Part model, mm, in its own coordinate system. A direction names the side the tool comes from. Give positions to 0.01 mm unless a question says otherwise; leave off trailing zeros. Order: outer loops, then holes, each group sorted by start corner. A loop starts at its lowest first (then second) coordinate and runs counter-clockwise, first axis right, second up. Notation, with made-up numbers: (-37.75, -17.75) - (-17.75, -17.75) arc R21 cw to (-17.75, -12.75) - close; hole circle Ø11 at (12, -16). An arc over 180 degrees is marked (long way). One line per item, written item: value.
```python
from build123d import *

# Parameters (mm, degrees)
RESSALTO_EXTRUS_O1_DEPTH = 10
CORTE_EXTRUS_O1_REACH    = 44.778
ESBO_O2_R                = 1.6
FILETE1_R                = 1.5
FILETE2_R                = 1.5
FILETE3_R                = 1.5


# Some blends are built 0.0001 mm under size
with BuildPart() as part:
    # Esboço1 → Ressalto-extrusão1 (new body)
    with BuildSketch(Plane.XY):
        Polygon((-37, -3), (-20, -3), (-20, 0), (-31, 0), (-31, 13), (31, 13), (31, 0), (20, 0), (20, -3), (37, -3), (37, 19), (-37, 19), align=None)
    extrude(amount=RESSALTO_EXTRUS_O1_DEPTH)

    # Esboço2 → Corte-extrusão1 (cut, up to next)
    with BuildSketch(Plane(origin=(0, 0, 0), x_dir=(1, 0, 0), z_dir=(0, 1, 0)), mode=Mode.PRIVATE) as corte_extrus_o1_sk1:
        with Locations(Location((-25.5, -5, 0), (0, 0, 180))):
            Circle(ESBO_O2_R)
    corte_extrus_o1_tool1 = extrude(corte_extrus_o1_sk1.sketch, amount=-CORTE_EXTRUS_O1_REACH, mode=Mode.PRIVATE) & part.part
    # Esboço2 → Corte-extrusão1 (cut, up to next)
    with BuildSketch(Plane(origin=(0, 0, 0), x_dir=(1, 0, 0), z_dir=(0, 1, 0)), mode=Mode.PRIVATE) as corte_extrus_o1_sk2:
        with Locations(Location((25.5, -5, 0), (0, 0, 270))):
            Circle(ESBO_O2_R)
    corte_extrus_o1_tool2 = extrude(corte_extrus_o1_sk2.sketch, amount=-CORTE_EXTRUS_O1_REACH, mode=Mode.PRIVATE) & part.part
    add(corte_extrus_o1_tool1.solids().sort_by_distance((-25.5, 0, 5))[0], mode=Mode.SUBTRACT)
    add(corte_extrus_o1_tool2.solids().sort_by_distance((25.5, 0, 5))[0], mode=Mode.SUBTRACT)

    # Filete1
    filete1_edges = [part.edges().sort_by_distance(p)[0] for p in [
        (0, 19, 0),
        (0, 13, 0),
        (0, 13, 10),
        (0, 19, 10),
    ]]
    fillet(filete1_edges, radius=FILETE1_R)

    # Filete2
    filete2_edges = [part.edges().sort_by_distance(p)[0] for p in [
        (37, 7.25, 10),
        (37, 18.560660172, 9.560660172),
        (37, 7.25, 0),
        (37, 18.560660172, 0.439339828),
        (-37, 7.25, 10),
        (-37, 18.560660172, 9.560660172),
        (-37, 7.25, 0),
        (-37, 18.560660172, 0.439339828),
        (37, 19, 5),
        (-37, 19, 5),
        (-20, -3, 5),
        (20, -3, 5),
        (-20, 0, 5),
        (20, 0, 5),
        (31, 0, 5),
        (-31, 0, 5),
        (-37, -3, 5),
        (37, -3, 5),
    ]]
    fillet(filete2_edges, radius=FILETE2_R - 0.0001)  # a hair under: the kernel refuses the full size

    # Filete3
    # the kernel refuses this fillet: 1.5 mm, written as the material it adds along each edge
    with BuildSketch(Plane(origin=(31, 13, 1.5), x_dir=(0, -1, 0), z_dir=(0, 0, 1))) as filete3_piece_1:
        with BuildLine():
            CenterArc((FILETE3_R, -FILETE3_R), FILETE3_R, 90, 90)
            Line((0, -FILETE3_R), (0, 0))
            Line((0, 0), (FILETE3_R, 0))
        make_face()
    extrude(amount=7)
    with BuildSketch(Plane(origin=(-31, 13, 1.5), x_dir=(0, -1, 0), z_dir=(0, 0, 1))) as filete3_piece_2:
        with BuildLine():
            CenterArc((FILETE3_R, FILETE3_R), FILETE3_R, 180, 90)
            Line((0, FILETE3_R), (0, 0))
            Line((0, 0), (FILETE3_R, 0))
        make_face()
    extrude(amount=7)
    with BuildSketch(Plane(origin=(31, 14.5, 8.5), x_dir=(0, 0.5976672776328287, -0.8017442392976475), z_dir=(0, -0.8017442392976475, -0.5976672776328287))) as filete3_piece_3_section:
        with BuildLine():
            CenterArc((1.5 + FILETE3_R, -FILETE3_R), FILETE3_R, 90, 90)
            Line((1.5, -FILETE3_R), (1.5, 0))
            Line((1.5, 0), (1.5 + FILETE3_R, 0))
        make_face()
    filete3_piece_3 = revolve(axis=Axis((31, 14.5, 8.5), (1, 0, 0)), revolution_arc=233.296989237, mode=Mode.PRIVATE)
    filete3_piece_3 = split(filete3_piece_3, bisect_by=Plane(origin=(30.532557549, 13.375091575, 10), z_dir=(0, 0, -1)), keep=Keep.TOP, mode=Mode.PRIVATE)
    add(filete3_piece_3)
    with BuildSketch(Plane(origin=(-31, 14.5, 8.5), x_dir=(0, 0.5976672776328287, -0.8017442392976475), z_dir=(0, -0.8017442392976475, -0.5976672776328287))) as filete3_piece_4_section:
        with BuildLine():
            CenterArc((1.5 + FILETE3_R, FILETE3_R), FILETE3_R, 180, 90)
            Line((1.5, FILETE3_R), (1.5, 0))
            Line((1.5, 0), (1.5 + FILETE3_R, 0))
        make_face()
    filete3_piece_4 = revolve(axis=Axis((-31, 14.5, 8.5), (1, 0, 0)), revolution_arc=233.296989237, mode=Mode.PRIVATE)
    filete3_piece_4 = split(filete3_piece_4, bisect_by=Plane(origin=(-30.532557659, 13.37509149, 10), z_dir=(0, 0, -1)), keep=Keep.TOP, mode=Mode.PRIVATE)
    add(filete3_piece_4)
    with BuildSketch(Plane(origin=(31, 14.5, 1.5), x_dir=(0, 0.5976672776328277, 0.8017442392976482), z_dir=(0, -0.8017442392976482, 0.5976672776328277))) as filete3_piece_5_section:
        with BuildLine():
            CenterArc((1.5 + FILETE3_R, FILETE3_R), FILETE3_R, 180, 90)
            Line((1.5, FILETE3_R), (1.5, 0))
            Line((1.5, 0), (1.5 + FILETE3_R, 0))
        make_face()
    filete3_piece_5 = revolve(axis=Axis((31, 14.5, 1.5), (-1, 0, 0)), revolution_arc=233.296989237, mode=Mode.PRIVATE)
    filete3_piece_5 = split(filete3_piece_5, bisect_by=Plane(origin=(30.532557549, 13.375091575, 0), z_dir=(0, 0, 1)), keep=Keep.TOP, mode=Mode.PRIVATE)
    add(filete3_piece_5)
    with BuildSketch(Plane(origin=(-31, 14.5, 1.5), x_dir=(0, 0.5976672776328277, 0.8017442392976482), z_dir=(0, -0.8017442392976482, 0.5976672776328277))) as filete3_piece_6_section:
        with BuildLine():
            CenterArc((1.5 + FILETE3_R, -FILETE3_R), FILETE3_R, 90, 90)
            Line((1.5, -FILETE3_R), (1.5, 0))
            Line((1.5, 0), (1.5 + FILETE3_R, 0))
        make_face()
    filete3_piece_6 = revolve(axis=Axis((-31, 14.5, 1.5), (-1, 0, 0)), revolution_arc=233.296989237, mode=Mode.PRIVATE)
    filete3_piece_6 = split(filete3_piece_6, bisect_by=Plane(origin=(-30.532557571, 13.375091573, 0), z_dir=(0, 0, 1)), keep=Keep.TOP, mode=Mode.PRIVATE)
    add(filete3_piece_6)


solid = part.part
```
1) Cut at A-A, the plane x = 25.5. Give the cut face in (y, z).
Outcome:
outline: (-3, 0) - (0, 0) - (0, 3.4) - (-3, 3.4) - close; (-3, 6.6) - (0, 6.6) - (0, 10) - (-3, 10) - close; (13, 1.5) arc R1.5 ccw to (14.5, 0) - (17.5, 0) arc R1.5 ccw to (19, 1.5) - (19, 8.5) arc R1.5 ccw to (17.5, 10) - (14.5, 10) arc R1.5 ccw to (13, 8.5) - close
2) Cut at B-B, the plane y = 8.75. Give the cut face in (x, z).
Outcome:
outline: (-37, 1.5) arc R1.5 ccw to (-35.5, 0) - (-31, 0) - (-31, 10) - (-35.5, 10) arc R1.5 ccw to (-37, 8.5) - close; (31, 0) - (35.5, 0) arc R1.5 ccw to (37, 1.5) - (37, 8.5) arc R1.5 ccw to (35.5, 10) - (31, 10) - close
3) Cut at C-C, the plane z = 5. Give the number of separate pieces and of enclosed holes in the cut face, then the cut area to 3 significant figures.
Outcome:
separate pieces: 3
enclosed holes: 0
area: 681 mm^2
4) Cut at D-D, the plane x = -18. Give the cut face in (y, z).
Outcome:
outline: (13, 1.5) arc R1.5 ccw to (14.5, 0) - (17.5, 0) arc R1.5 ccw to (19, 1.5) - (19, 8.5) arc R1.5 ccw to (17.5, 10) - (14.5, 10) arc R1.5 ccw to (13, 8.5) - close
5) Pin check, flat tips, straight feed: pin 1 (1 mm diameter, centred on x = 16.5, z = 4, fed in from -Y); pin 2 (5 mm diameter, centred on x = -3, y = 11, fed in from +Z); pin 3 (8 mm diameter, centred on x = 7.5, y = 14, fed in from +Z). Stop position of each tip, or through.
Outcome:
pin 1: stops at y = 13
pin 2: stops at z = 9.62
pin 3: stops at z = 10
6) Drill centre lines: line 1 along X through (y, z) = (11.25, 5); line 2 along Y through (x, z) = (22, 4.5); line 3 along Z through (x, y) = (-25.5, -1.2). Where is each one in solid material? Low to high. Write a range as from..to.
Outcome:
line 1: x = -37..-31, 31..37
line 2: y = -3..0, 13..19
line 3: z = 0..3.4, 6.6..10
7) Which spindle directions (+Z, -Z, +X, -X, +Y, -Y) get a long thin tool onto all of the face, cutting with end or side? Do faces 5 (the cylindrical face through (0.41, 13.45, 9.57)), 6 (the cylindrical face through (-30.55, 0.43, 5.07)), 7 (the flat face through (-29, -3, 5)), 8 (the cylindrical face through (20.45, -2.57, 5.07)), 9 (the cylindrical face through (25.981, -1.479, 6.526)). Say none if no direction does.
Outcome:
face 5: +Z
face 6: +Z, -Z
face 7: +Z, -Z, +X, -X, -Y
face 8: +Z, -Z, -Y
face 9: -Y
8) Mould opens along X. For faces 1 (the cylindrical face through (-0.5, 18.55, 0.43)), 2 (the cylindrical face through (-36.57, 7.39, 0.45)), 3 (the cylindrical face through (30.57, 12.55, 4.95)), 4 (the cylindrical face through (36.57, 7.11, 0.45)) say: released by +X, released by -X, zero draft, split by the parting line, or undercut.
Outcome:
face 1: zero draft
face 2: released by -X
face 3: undercut
face 4: released by +X
